Could you check a few things on this model? Use its own coordinates, in mm. Face numbers are marked on the shaded views. A direction names the side the tool comes from. Give positions to 0.01 mm unless a question says otherwise; leave off trailing zeros. Loops run counter-clockwise (first coordinate to the right, second up) from the corner with the lowest first, then second, coordinate; pieces in that order, holes last. Notation, with made-up numbers: M 32,61 L 79,61 A13 ccw 79,66 Z; hole C 10,79 d3. An arc over 180 degrees is marked long. Answer in a Markdown table with one row per item. Add a question column.
Autodesk Fusion 360 part; units mm, degrees
sketch "Sketch1" plane through (0, 0, 0) normal (0, 1, 0) x (1, 0, 0)
  line L0 (48, 20) -> (-48, 20)
  line L1 (-48, 20) -> (-48, -20)
  line L2 (-48, -20) -> (48, -20)
  line L3 (48, -20) -> (48, 20)
  line L4 (48, 20) -> (-48, -20) construction
  line L5 (-48, 20) -> (48, -20) construction
  line L6 (47.25, 19.25) -> (-47.25, 19.25)
  line L7 (-47.25, 19.25) -> (-47.25, -19.25)
  line L8 (-47.25, -19.25) -> (47.25, -19.25)
  line L9 (47.25, -19.25) -> (47.25, 19.25)
  line L10 (47.25, 19.25) -> (-47.25, -19.25) construction
  line L11 (-47.25, 19.25) -> (47.25, -19.25) construction
  dimension "d1" = 96
  dimension "d2" = 40
  dimension "d3" = 94.5
  dimension "d4" = 38.5
extrude "Extrude1" add sketch "Sketch1" along normal blind 14
sketch "Sketch2" plane through (0, 0, 0) normal (0, 1, 0) x (1, 0, 0)
  line L0 (-48, -20) -> (48, -20)
  line L1 (48, -20) -> (48, 20)
  line L2 (48, 20) -> (-48, 20)
  line L3 (-48, 20) -> (-48, -20)
extrude "Extrude2" add sketch "Sketch2" against normal blind 1.5
sketch "Sketch3" plane through (0, -1.5, 0) normal (0, -1, 0) x (1, 0, 0)
  line L0 (-48, 20) -> (-48, -20)
  line L1 (-48, -20) -> (48, -20)
  line L2 (48, -20) -> (48, 20)
  line L3 (48, 20) -> (-48, 20)
  circle A0 centre (-40.3833, 13.3405) radius 2.5
  dimension "d10" = 5
extrude "Extrude3" cut sketch "Sketch3" against normal blind 2.918 contours A0
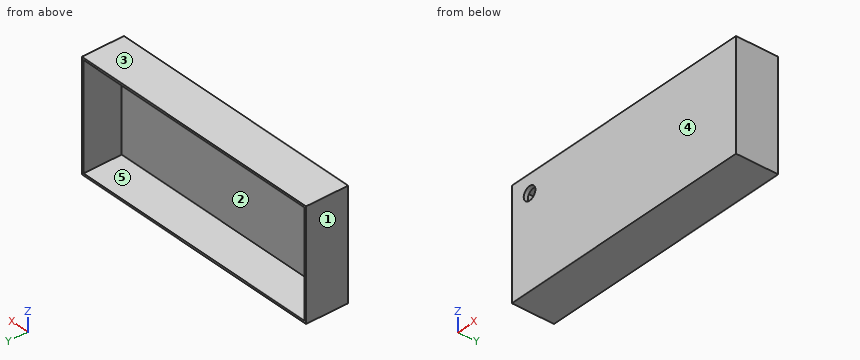
Item 1: For P1, Ø4.5, axis at x = -40.38, z = 13.34, coming from the +Y side; P2, Ø2, axis at x = -11.5, z = 12.5, coming from the +Y side, each with a flat end and sliding along its axis, tell me the tip position at first contact or that it passes through.
Item 2: If we mould it in two halves opening along X, with no side actions, what happens to the marked faces 1, 2 and 3? For each: +X half, -X half, draft (parallel to the pull), parting line (faces both ways), or undercut.
Item 3: Suppose I cut it at C-C (x = -3). List the corners of the cut face in (y, z) for me, then the cut area to 3 significant figures.
Item 4: Suppose I cut it at B-B (z = 9). List the corners of the cut face in (x, y) for me.
Item 5: For the marked faces 4 and 5, which set-ups out of +Z, -Z, +X, -X, +Y, -Y let a thin tool reach every point of the face, with its end or its side?
Item 6: Suppose I cut it at A-A (y = 10). List the corners of the cut face in (x, z) for me, then the cut area to 3 significant figures.
Item 7: I need wall thicknesses on L1, parallel to Z at x = -4, y = 6.25; L2, parallel to X at y = 0.25, z = 6; L3, parallel to Y at x = 6.5, z = 5. Which ranges of each line are inside material? Lowest first, please.
Values found:
| question | item | result |
|---|---|---|
| 1 | P1 | through |
| 1 | P2 | y = 0 |
| 2 | face 1 | -X half |
| 2 | face 2 | undercut |
| 2 | face 3 | draft |
| 3 | outline | M -1.5,-20 L 14,-20 L 14,-19.25 L 0,-19.25 L 0,19.25 L 14,19.25 L 14,20 L -1.5,20 Z |
| 3 | area | 81.0 mm² |
| 4 | outline | M -48,-1.5 L 48,-1.5 L 48,14 L 47.25,14 L 47.25,0 L -47.25,0 L -47.25,14 L -48,14 Z |
| 5 | face 4 | +Z, -Z, +X, -X, -Y |
| 5 | face 5 | +Y |
| 6 | outline | M -48,-20 L 48,-20 L 48,20 L -48,20 Z; hole M -47.25,-19.25 L 47.25,-19.25 L 47.25,19.25 L -47.25,19.25 Z |
| 6 | area | 202 mm² |
| 7 | L1 | -20 to -19.25, 19.25 to 20 |
| 7 | L2 | -48 to -47.25, 47.25 to 48 |
| 7 | L3 | -1.5 to 0 |
